from build123d import *

# Parameters (mm, degrees)
SKETCH1_R               = 76.2
EXTRUDE1_DEPTH          = 75.946
SKETCH2_R               = 127
EXTRUDE2_DEPTH          = 24.638
CUT_EXTRUDE1_DEPTH      = 196.002038236
CUT_EXTRUDE1_DEPTH_BACK = 65.9384
SKETCH3_R               = 74.168
SKETCH4_R               = 50.8
CUT_EXTRUDE2_DEPTH      = 196.002038236
CIRPATTERN2_COUNT       = 16
SKETCH5_R               = 4.2164
CUT_EXTRUDE5_DEPTH      = 196.002038236
CIRPATTERN3_COUNT       = 24


with BuildPart() as part:
    # Sketch1 → Extrude1 (new body)
    with BuildSketch(Plane(origin=(0, 0, 0), x_dir=(1, 0, 0), z_dir=(0, 1, 0))):
        with Locations(Location((0, 0, 0), (0, 0, 270))):
            Circle(SKETCH1_R)
    extrude(amount=-EXTRUDE1_DEPTH)

    # Sketch2 → Extrude2 (add)
    with BuildSketch(Plane(origin=(0, 0, 0), x_dir=(1, 0, 0), z_dir=(0, 1, 0))):
        with Locations(Location((0, 0, 0), (0, 0, 90))):
            Circle(SKETCH2_R)
    extrude(amount=EXTRUDE2_DEPTH)

    # Sketch3 → Cut-Extrude1 (cut, two sides: drawn at the far end of the back side and taken through both)
    with BuildSketch(Plane(origin=(0, 0, 0), x_dir=(1, 0, 0), z_dir=(0, 1, 0)).offset(-CUT_EXTRUDE1_DEPTH_BACK)):
        with Locations(Location((0, 0, 0), (0, 0, 90))):
            Circle(SKETCH3_R)
    extrude(amount=CUT_EXTRUDE1_DEPTH + CUT_EXTRUDE1_DEPTH_BACK, mode=Mode.SUBTRACT)

    # Sketch4 → Cut-Extrude2 (cut, through all)
    with BuildSketch(Plane(origin=(0, 0, 0), x_dir=(1, 0, 0), z_dir=(0, 1, 0))):
        with Locations(Location((0, 0, 0), (0, 0, 270))):
            Circle(SKETCH4_R)
    extrude(amount=-CUT_EXTRUDE2_DEPTH, mode=Mode.SUBTRACT)

    # Sketch11 → 1/4-20 Tapped Hole1 (revolve, cut)
    with BuildSketch(Plane(origin=(0, 24.638, -85.725), x_dir=(0, 0, 1), z_dir=(1, 0, 0))):
        Polygon((0, 0), (0, 18.043816902), (2.5527, 16.51), (2.5527, 0), align=None)
    f_1_4_20_tapped_hole1 = revolve(axis=Axis((0, 30.988, -85.725), (0, -1, 0)), mode=Mode.SUBTRACT)

    # CirPattern2: 1/4-20 Tapped Hole1 ×16 about axis
    cirpattern2_axis = Axis((0, 0, 0), (0, 1, 0))
    for i in range(1, CIRPATTERN2_COUNT):
        add(f_1_4_20_tapped_hole1.rotate(cirpattern2_axis, i * 360 / CIRPATTERN2_COUNT), mode=Mode.SUBTRACT)

    # Sketch5 → Cut-Extrude5 (cut, through all)
    with BuildSketch(Plane(origin=(0, 0, 0), x_dir=(1, 0, 0), z_dir=(0, 1, 0))):
        with Locations(Location((-15.134642514, 114.959023121, 0), (0, 0, 90))):
            Circle(SKETCH5_R)
    cut_extrude5 = extrude(amount=CUT_EXTRUDE5_DEPTH, mode=Mode.SUBTRACT)

    # CirPattern3: Cut-Extrude5 ×24 about axis
    cirpattern3_axis = Axis((0, 0, 0), (0, 1, 0))
    for i in range(1, CIRPATTERN3_COUNT):
        add(cut_extrude5.rotate(cirpattern3_axis, i * 360 / CIRPATTERN3_COUNT), mode=Mode.SUBTRACT)


solid = part.part
CAD build for the part. Positions are in the model's coordinates, mm. A direction names the side the tool comes from. Coordinates: 2 decimals unless noted, no trailing zeros. Order: outer loops, then holes, each group sorted by start corner. A loop starts at its lowest first (then second) coordinate and runs counter-clockwise, first axis right, second up. Notation, with made-up numbers: (0.5, -4.75) -> (17.5, -4.75) arc R19 ccw to (17.5, 30.25) -> close; hole circle Ø8 at (-11, 8). An arc over 180 degrees is marked (long way). Answer in a Markdown table with one row per item.
1) Mould opens along X. For faces 1 (the face through (-47.48, 12.147, 104.275)), 2 (the face through (55, 0, -55)), 3 (the face through (123.98, 12.15, 27.53)) say: pulls with the +X half, pulls with the -X half, needs draft (parallel to the pull), parting line crosses it, or undercut.
Check values:
| item | result |
|---|---|
| face 1 | undercut |
| face 2 | needs draft |
| face 3 | parting line crosses it |
2) Band-saw the part on C-C (x = -26.5). List the corners of the cut face in (y, z), and give its area (3 significant figures).
Check values:
| item | result |
|---|---|
| outline | (-75.95, -71.44) -> (0, -71.44) -> (0, -124.2) -> (24.64, -124.2) -> (24.64, -69.27) -> (-65.94, -69.27) -> (-65.94, -43.34) -> (-75.95, -43.34) -> close; (-75.95, 43.34) -> (-65.94, 43.34) -> (-65.94, 69.27) -> (24.64, 69.27) -> (24.64, 124.2) -> (0, 124.2) -> (0, 71.44) -> (-75.95, 71.44) -> close |
| area | 3,560 mm2 |
3) Band-saw the part on B-B (y = -37.5). List the corners of the cut face in (x, z), and give its area (3 significant figures).
Check values:
| item | result |
|---|---|
| outline | circle Ø152.4 at (0, 0); hole circle Ø148.34 at (0, 0) |
| area | 960 mm2 |
4) Band-saw the part on A-A (z = -7). List the corners of the cut face in (x, y).
Check values:
| item | result |
|---|---|
| outline | (-126.81, 0) -> (-75.88, 0) -> (-75.88, -75.95) -> (-50.32, -75.95) -> (-50.32, -65.94) -> (-73.84, -65.94) -> (-73.84, 24.64) -> (-126.81, 24.64) -> close; (50.32, -75.95) -> (75.88, -75.95) -> (75.88, 0) -> (126.81, 0) -> (126.81, 24.64) -> (73.84, 24.64) -> (73.84, -65.94) -> (50.32, -65.94) -> close |
5) Drill centre lines: line 1 (X direction, y = 15, z = 106); line 2 (Y direction, x = 14, z = 97.5); line 3 (Z direction, x = 78.5, y = 17.5). Where is each one in solid material? Low to high.
Check values:
| item | result |
|---|---|
| line 1 | -69.95 to -48.44, -40.31 to 40.31, 48.44 to 69.95 |
| line 2 | 0 to 24.64 |
| line 3 | -99.83 to -35.26, -30.35 to 30.35, 35.26 to 99.83 |
6) Which spindle directions (+Z, -Z, +X, -X, +Y, -Y) get a long thin tool onto all of the face, cutting with end or side? Do faces 4 (the face through (-46.367, -37.441, -60.47)), 5 (the face through (104.557, 12.147, -41.028)), 6 (the face through (48, -65.938, 18)). Say none if no direction does.
Check values:
| item | result |
|---|---|
| face 4 | -Y |
| face 5 | +Y, -Y |
| face 6 | +Y |
7) Flat gauge pins, fed straight in: P1, Ø6, axis at y = -64, z = -3, coming from the +X side; P2, Ø4, axis at x = -69.5, y = -13.5, coming from the -Z side; P3, Ø6, axis at x = 60.62, z = -60.62, coming from the -Y side. Where does each tip first touch, or does it go through?
Check values:
| item | result |
|---|---|
| P1 | x = 76.2 |
| P2 | z = -35.36 |
| P3 | y = 0 |
